Here's how the part is built. I have some questions about the finished solid (model axes, mm). Face numbers are marked on the shaded views. Round coordinates to 2 decimals unless told otherwise and drop trailing zeros. Order: outer loops, then holes, each group sorted by start corner. A loop starts at its lowest first (then second) coordinate and runs counter-clockwise, first axis right, second up. Notation, with made-up numbers: M 32.25,-40 L 45.25,-40 A17 ccw 45.25,-27 Z; hole C 63,50.5 d7. An arc over 180 degrees is marked long. Use one line per item in the form item = value. Start each with the question number.
```python
from build123d import *

# Parameters (mm, degrees)
EXTRUDE_1_DEPTH          = 15
CUT_EXTRUDE_1_DEPTH      = 28.393120676
CUT_EXTRUDE_1_DEPTH_BACK = 28.393120676
SKETCH_2_R               = 1.6


with BuildPart() as part:
    # 草图1 → 凸台-拉伸1 (new body)
    with BuildSketch(Plane.XY):
        with BuildLine():
            Line((-18.631868928, -12.71063098), (-18.925857281, -12.705463728))
            Line((-18.925857281, -12.705463728), (-18.925857281, -15.71063098))
            Line((-18.925857281, -15.71063098), (19.074142719, -15.71063098))
            Line((19.074142719, -15.71063098), (19.074142719, -12.71063098))
            Line((19.074142719, -12.71063098), (5.86854838, -12.71063098))
            ThreePointArc((5.86854838, -12.71063098), (11.79321155, -7.544545138), (14, 0))
            Line((14, 0), (10, 0))
            ThreePointArc((10, 0), (0, -10), (-10, 0))
            Line((-10, 0), (-14, 0))
            ThreePointArc((-14, 0), (-11.79321155, -7.544545138), (-5.86854838, -12.71063098))
            Line((-5.86854838, -12.71063098), (-18.631868928, -12.71063098))
        make_face()
    extrude(amount=EXTRUDE_1_DEPTH)

    # 草图2 → 切除-拉伸1 (cut, two sides: drawn at the far end of the back side and taken through both)
    with BuildSketch(Plane(origin=(0, -12.71063098, 0), x_dir=(1, 0, 0), z_dir=(0, 1, 0)).offset(-CUT_EXTRUDE_1_DEPTH_BACK)):
        with Locations(Location((-13.190081146, -9, 0), (0, 0, 180))):
            Circle(SKETCH_2_R)
        with Locations(Location((12.809918854, -9, 0), (0, 0, 180))):
            Circle(SKETCH_2_R)
    extrude(amount=CUT_EXTRUDE_1_DEPTH + CUT_EXTRUDE_1_DEPTH_BACK, mode=Mode.SUBTRACT)


solid = part.part
```
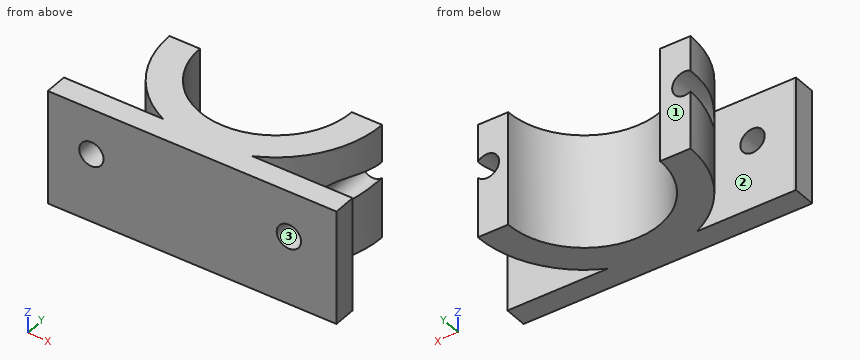
1) If I drill on line 1 (X direction, y = -14.35, z = 9); line 2 (X direction, y = -3.5, z = 9); line 3 (Y direction, x = 8, z = 10), over which ranges is the centre line in solid material (lowest first)?
2) If we section it at A-A on z = 9: Write out the boundary of the cut face in (x, y).
3) If we section it at C-C on y = -14.5: Write out the boundary of the cut face in (x, z), then the cut area to 3 significant figures.
4) If we section it at D-D on z = 11.5: Write out the boundary of the cut face in (x, y).
5) Will these pins go through, and if not, where does the flat tip stop? pin 1 Ø2 at (x, z) = (-5, 7.5) entering from +Y; pin 2 Ø2 at (y, z) = (-5.5, 10.5) entering from +X; pin 3 Ø6 at (y, z) = (-8.5, 2.5) entering from -X; pin 4 Ø2.5 at (x, z) = (12.81, 9) entering from -Y.
6) If we mould it in two halves opening along Y, with no side actions, what happens to the marked faces 1, 2 and 3? For each: +Y half, -Y half, draft (parallel to the pull), parting line (faces both ways), or undercut.
7) If we section it at B-B on x = 9.5: Write out the boundary of the cut face in (y, z).
Completed:
q1.line_1 = -18.93 to -14.79, -11.59 to 11.21, 14.41 to 19.07
q1.line_2 = -11.59 to -9.37, 9.37 to 11.21
q1.line_3 = -15.71 to -12.71, -11.49 to -6
q2.outline = M -18.93,-15.71 L -14.79,-15.71 L -14.79,-12.71 L -18.63,-12.71 L -18.93,-12.71 Z; M -11.59,-15.71 L 11.21,-15.71 L 11.21,-12.71 L 5.87,-12.71 A14 ccw 11.21,-8.39 L 11.21,0 L 10,0 A10 cw -10,0 L -11.59,0 L -11.59,-7.85 A14 ccw -5.87,-12.71 L -11.59,-12.71 Z; M 14.41,-15.71 L 19.07,-15.71 L 19.07,-12.71 L 14.41,-12.71 Z
q3.outline = M -18.93,0 L 19.07,0 L 19.07,15 L -18.93,15 Z; hole C -13.19,9 d3.2; hole C 12.81,9 d3.2
q3.area = 554 mm²
q4.outline = M -18.93,-15.71 L 19.07,-15.71 L 19.07,-12.71 L 5.87,-12.71 A14 ccw 14,0 L 10,0 A10 cw -10,0 L -14,0 A14 ccw -5.87,-12.71 L -18.63,-12.71 L -18.93,-12.71 Z
q5.pin_1 = -8
q5.pin_2 = 13.26
q5.pin_3 = -12.87
q5.pin_4 = through
q6.face_1 = +Y half
q6.face_2 = undercut
q6.face_3 = draft
q7.outline = M -15.71,0 L -12.71,0 L -12.71,15 L -15.71,15 Z; M -10.28,0 L -3.12,0 L -3.12,15 L -10.28,15 Z
